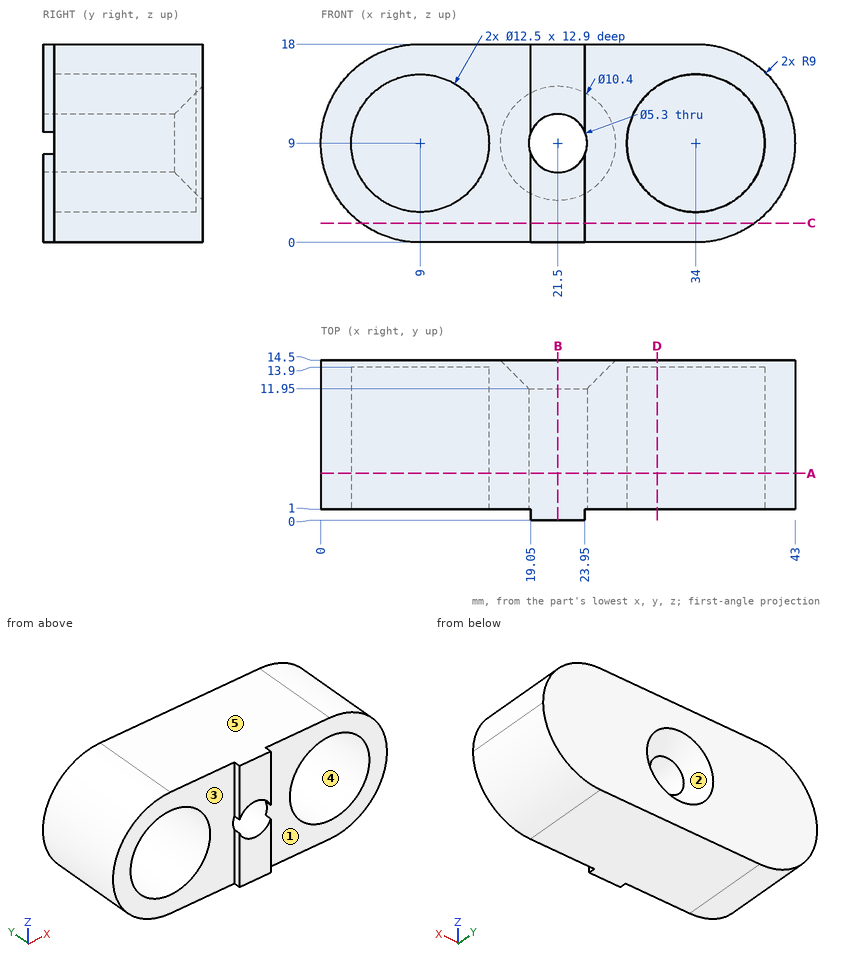
The figure shows three views and two pictorial views of one solid part (mm, origin at its lowest corner). Answer the questions. A direction names the side the tool comes from. Give positions to 0.01 mm unless a question says otherwise; leave off trailing zeros. Order: outer loops, then holes, each group sorted by start corner. A loop starts at its lowest first (then second) coordinate and runs counter-clockwise, first axis right, second up. Notation, with made-up numbers: (23.25, 76.5) -> (31.25, 76.5) arc R34 cw to (31.25, 112.5) -> close; hole circle Ø5 at (76.5, 28). An arc over 180 degrees is marked (long way). One line per item, written item: value.
1) Find the intervals of material crossed by line 1 (X direction, y = 8.25, z = 9); line 2 (Z direction, x = 34, y = 13.5); line 3 (X direction, y = 10, z = 12.75), in increasing order.
Reported:
line 1: x = 0 to 2.75, 15.25 to 18.85, 24.15 to 27.75, 40.25 to 43
line 2: z = 0 to 2.75, 15.25 to 18
line 3: x = 0.82 to 4, 14 to 29, 39 to 42.18
2) Find section A-A, the plane y = 4.25. Determine the outline of the cut face in (x, z).
Reported:
outline: (9, 0) -> (34, 0) arc R9 ccw to (34, 18) -> (9, 18) arc R9 ccw to start; hole circle Ø12.5 at (9, 9); hole circle Ø5.3 at (21.5, 9); hole circle Ø12.5 at (34, 9)
3) Find section D-D, the plane x = 30.5. Determine the outline of the cut face in (y, z), plus the area to 3 significant figures.
Reported:
outline: (1, 0) -> (14.5, 0) -> (14.5, 18) -> (1, 18) -> (1, 14.18) -> (13.9, 14.18) -> (13.9, 3.82) -> (1, 3.82) -> close
area: 109 mm^2
4) A tool of negligible diameter and unlimited length cuts with its end or side. For the marked faces 1, 2, 3, 4 and 5, from which of +Z, -Z, +X, -X, +Y, -Y can it reach the whole face along a straight path? Write none if from no direction.
Reported:
face 1: +Z, -Z, +X, -Y
face 2: +Y
face 3: +Z, -Z, -X, -Y
face 4: -Y
face 5: +Z, +X, -X, +Y, -Y
5) Find section C-C, the plane z = 1.75. Determine the outline of the cut face in (x, y).
Reported:
outline: (3.67, 1) -> (19.05, 1) -> (19.05, 0) -> (23.95, 0) -> (23.95, 1) -> (39.33, 1) -> (39.33, 14.5) -> (3.67, 14.5) -> close
6) Find section B-B, the plane x = 21.5. Determine the outline of the cut face in (y, z), plus the area to 3 significant figures.
Reported:
outline: (0, 0) -> (14.5, 0) -> (14.5, 3.8) -> (11.95, 6.35) -> (0, 6.35) -> close; (0, 11.65) -> (11.95, 11.65) -> (14.5, 14.2) -> (14.5, 18) -> (0, 18) -> close
area: 178 mm^2
7) Flat-ended cylindrical pins translate along their axes: P1, Ø6, axis at x = 21.5, z = 9, coming from the +Y side; P2, Ø0.5, axis at y = 0.5, z = 15, coming from the -X side; P3, Ø10, axis at x = 35.5, z = 12, coming from the -Y side. Find the tip coordinate at first contact, or state that the pin passes through.
Reported:
P1: stops at y = 12.3
P2: stops at x = 19.05
P3: stops at y = 1
